Geometry: see drawing. Coordinates: mm, zero at the bounding-box minimum. A direction names the side the tool comes from. Coordinates: 2 decimals unless noted, no trailing zeros. Write each loop counter-clockwise with the first axis right and the second up, starting at its lowest first coordinate (ties: lowest second). Pieces come first, ordered by that corner, then holes.
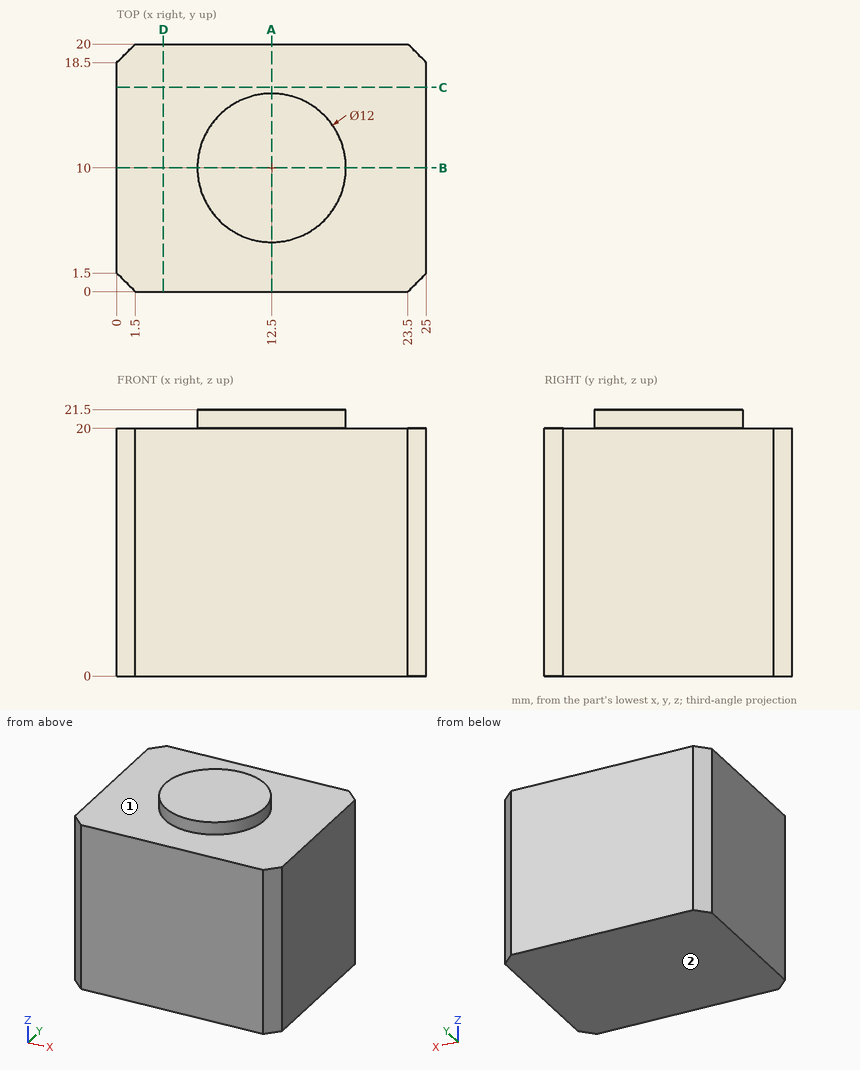
Item 1: Section B-B, the plane y = 10. Output: boundary loops of the cut face in (x, z), plus the area to 3 significant figures.
Derived:
outline: (0, 0) - (25, 0) - (25, 20) - (18.5, 20) - (18.5, 21.5) - (6.5, 21.5) - (6.5, 20) - (0, 20) - close
area: 518 mm2
Item 2: Set-up query: the marked faces 1 and 2. Return all of +Z, -Z, +X, -X, +Y, -Y with unobstructed straight access to the full face (end or side cutting, diameter ignored); none if empty.
Derived:
face 1: +Z
face 2: -Z, +X, -X, +Y, -Y
Item 3: Section C-C, the plane y = 16.5. Output: boundary loops of the cut face in (x, z), plus the area to 3 significant figures.
Derived:
outline: (0, 0) - (25, 0) - (25, 20) - (0, 20) - close
area: 500 mm2
Item 4: Section D-D, the plane x = 3.75. Output: boundary loops of the cut face in (y, z), plus the area to 3 significant figures.
Derived:
outline: (0, 0) - (20, 0) - (20, 20) - (0, 20) - close
area: 400 mm2
Item 5: Material intervals for probe 1 along Z at (x, y) = (21, 13.5); probe 2 along X at (y, z) = (19, 2.5), sorted ascending.
Derived:
probe 1: z = 0 to 20
probe 2: x = 0.5 to 24.5
Item 6: Pin query (flat end, axial travel): pin 1 (1 mm diameter, centred on x = 6, y = 6, fed in from +Z). Return the tip coordinate at first contact, or that it passes through.
Derived:
pin 1: stops at z = 20
Item 7: Section A-A, the plane x = 12.5. Output: boundary loops of the cut face in (y, z), plus the area to 3 significant figures.
Derived:
outline: (0, 0) - (20, 0) - (20, 20) - (16, 20) - (16, 21.5) - (4, 21.5) - (4, 20) - (0, 20) - close
area: 418 mm2
